Part model, mm, in its own coordinate system. Face numbers are marked on the shaded views. A direction names the side the tool comes from. Coordinates: 2 decimals unless noted, no trailing zeros. Order: outer loops, then holes, each group sorted by start corner. A loop starts at its lowest first (then second) coordinate and runs counter-clockwise, first axis right, second up. Notation, with made-up numbers: M 38.5,76.25 L 74.5,76.25 A13 cw 74.5,96.25 Z; hole C 63,31.25 d11. An arc over 180 degrees is marked long. Write item = value, one per line. Start each with the question number.
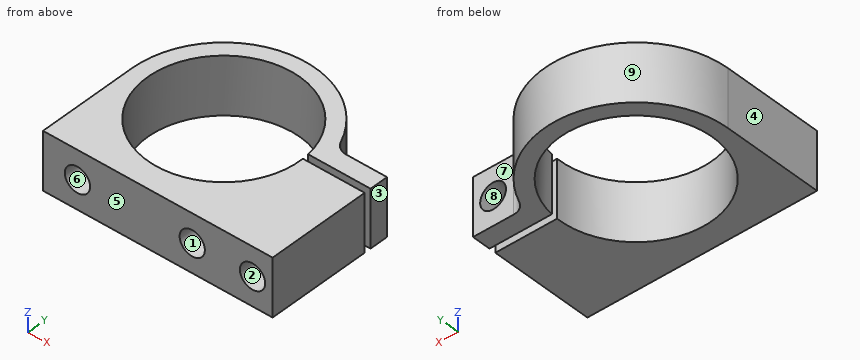
from build123d import *

# Parameters (mm, degrees)
F1_DEPTH  = 20
F2_R      = 26.5
F3_DEPTH  = 20
F4_W      = 50
F4_H      = 2.3
F5_DEPTH  = 20.001
F7_D      = 8.8
F7_DEPTH  = 12
F7_TIP    = 2.6437867237
F8_R      = 5
F10_D     = 8.8
F10_DEPTH = 36.2202316189
F11_D     = 9
F11_DEPTH = 30.7817683811


# Not quite as in the source:
# - a feature of the source that left no trace in its solid (it failed there, or was rolled back) is left out


with BuildPart() as f1:
    # F0 (on Top) → F1 (new body)
    with BuildSketch(Plane.XY):
        with BuildLine():
            ThreePointArc((30.3973683071, 27.5), (-5.0638036184, 49.0968019412), (-32, 17.5))
            Line((-32, 17.5), (-32, -17.5))
            Line((-32, -17.5), (48, -17.5))
            Line((48, -17.5), (48, 27.5))
            Line((48, 27.5), (30.3973683071, 27.5))
        make_face()
    extrude(amount=F1_DEPTH)

    # F2 (on face) → F3 (cut, through all)
    with BuildSketch(Plane.XY.offset(20)):
        with Locations((0, 17.5)):
            Circle(F2_R)
    extrude(amount=-F3_DEPTH, mode=Mode.SUBTRACT)

    # F4 (on face) → F5 (cut, through all)
    with BuildSketch(Plane.XY.offset(20)):
        with Locations((45, 19.8692316189)):
            Rectangle(F4_W, F4_H)
    extrude(amount=-F5_DEPTH, mode=Mode.SUBTRACT)

    # F7
    with Locations(Plane.XZ.offset(17.5)):
        with Locations((-20, 10), (20, 10)):
            Hole(F7_D / 2, depth=F7_DEPTH)
            with Locations((0, 0, -(F7_DEPTH + F7_TIP / 2))):  # 118° drill point
                Cone(0, F7_D / 2, F7_TIP, mode=Mode.SUBTRACT)

    # F8
    f8_edges = [f1.edges().sort_by_distance(p)[0] for p in [
        (30.397368, 27.5, 10),
    ]]
    fillet(f8_edges, radius=F8_R)

    # F10 (through all, one way)
    with BuildSketch(Plane(origin=(0, 18.7192316189, 0), x_dir=(-1, 0, 0), z_dir=(0, 1, 0))):
        with Locations((-41, 10)):
            Circle(F10_D / 2)
    extrude(amount=-F10_DEPTH, mode=Mode.SUBTRACT)

    # F11 (through all, one way)
    with BuildSketch(Plane(origin=(0, 18.7192316189, 0), x_dir=(-1, 0, 0), z_dir=(0, -1, 0))):
        with Locations((-41, -10)):
            Circle(F11_D / 2)
    extrude(amount=-F11_DEPTH, mode=Mode.SUBTRACT)


solid = f1.part
Item 1: 3-axis set-ups, long thin cutter, end or side, ignore diameter. For the marked faces 5, 6, 7, 8 and 9: which of +Z, -Z, +X, -X, +Y, -Y reach the whole face in a straight line?
Item 2: Cut at A-A, the plane x = 41. Write the cut outline in (y, z).
Item 3: Wall check: line 1 along Z through (x, y) = (41, 3.5); line 2 along X through (y, z) = (12, 12.75); line 3 along Z through (x, y) = (41, 24). Give the ranges that are in metal, low to high. Write a range as [from, to].
Item 4: Cut at D-D, the plane z = 3.25. Write the cut outline in (x, y), and give its area (3 significant figures).
Item 5: Cut at C-C, the plane x = 0. Write the cut outline in (y, z), and give its area (3 significant figures).
Item 6: Flat gauge pins, fed straight in: pin 1 (5.5 mm diameter, centred on x = 20, z = 10, fed in from +Y); pin 2 (12 mm diameter, centred on x = -18, y = 36, fed in from +Z); pin 3 (2 mm diameter, centred on y = 39.5, z = 5.5, fed in from +X); pin 4 (5 mm diameter, centred on x = -3, z = 6.5, fed in from +Y). Where does each tip first touch, or does it go through?
Item 7: Pull direction X, two halves, no side cores. Call the marked faces 1, 2, 3 and 4: pulls with the +X half, pulls with the -X half, needs draft (parallel to the pull), parting line crosses it, or undercut.
Item 8: Cut at B-B, the plane y = 39.5. Write the cut outline in (x, z).
Filled sheet:
q1.face_5 = +Z, -Z, +X, -X, -Y
q1.face_6 = -Y
q1.face_7 = +Z, -Z, +X, +Y
q1.face_8 = +Y
q1.face_9 = +Z, -Z, +Y
q2.outline = M -17.5,0 L 18.72,0 L 18.72,5.6 L -17.5,5.6 Z; M -17.5,14.4 L 18.72,14.4 L 18.72,20 L -17.5,20 Z; M 21.02,0 L 27.5,0 L 27.5,5.5 L 21.02,5.5 Z; M 21.02,14.5 L 27.5,14.5 L 27.5,20 L 21.02,20 Z
q3.line_1 = [0, 5.6], [14.4, 20]
q3.line_2 = [-32, -25.92], [25.92, 37.57], [44.43, 48]
q3.line_3 = [0, 5.5], [14.5, 20]
q4.outline = M -32,-17.5 L 48,-17.5 L 48,18.72 L 26.47,18.72 A26.5 cw long 26.27,21.02 L 48,21.02 L 48,27.5 L 33.82,27.5 A5 cw 29.25,30.47 A32 ccw -32,17.5 Z
q4.area = 2,320 mm2
q5.outline = M -17.5,0 L -9,0 L -9,20 L -17.5,20 Z; M 44,0 L 49.5,0 L 49.5,20 L 44,20 Z
q5.area = 280 mm2
q6.pin_1 = 44.45
q6.pin_2 = 20
q6.pin_3 = 24.15
q6.pin_4 = 49.5
q7.face_1 = undercut
q7.face_2 = undercut
q7.face_3 = pulls with the +X half
q7.face_4 = pulls with the -X half
q8.outline = M -23.24,0 L -14.77,0 L -14.77,20 L -23.24,20 Z; M 14.77,0 L 23.24,0 L 23.24,20 L 14.77,20 Z
